from build123d import *

# Parameters (mm, degrees)
SKETCH3_W               = 130
SKETCH3_H               = 45
BOSS_EXTRUDE1_DEPTH     = 100
CUT_EXTRUDE1_DEPTH      = 122.372360939
CUT_EXTRUDE1_DEPTH_BACK = 122.372360939
BOSS_EXTRUDE2_DEPTH     = 8
CUT_EXTRUDE2_DEPTH      = 122.372360939
CUT_EXTRUDE2_DEPTH_BACK = 122.372360939
CUT_EXTRUDE3_DEPTH      = 122.372360939
CUT_EXTRUDE3_DEPTH_BACK = 122.372360939
CUT_EXTRUDE4_DEPTH      = 122.372360939
CUT_EXTRUDE4_DEPTH_BACK = 122.372360939
FILLET3_R               = 5
SKETCH16_R              = 10
SKETCH16_R_2            = 5
BOSS_EXTRUDE3_DEPTH     = 15
SKETCH19_R              = 6
CUT_EXTRUDE5_DEPTH      = 122.372360939
CUT_EXTRUDE6_DEPTH      = 147.735305908
CUT_EXTRUDE6_DEPTH_BACK = 147.735305908
SKETCH23_R              = 5
CUT_EXTRUDE7_DEPTH      = 15
CUT_EXTRUDE8_DEPTH      = 15
CUT_EXTRUDE9_DEPTH      = 166.548331311
CUT_EXTRUDE9_DEPTH_BACK = 166.548331311
SKETCH28_R              = 11


with BuildPart() as part:
    # Sketch3 → Boss-Extrude1 (new body)
    with BuildSketch(Plane(origin=(0, 0, 0), x_dir=(1, 0, 0), z_dir=(0, 1, 0))):
        Rectangle(SKETCH3_W, SKETCH3_H)
    extrude(amount=-BOSS_EXTRUDE1_DEPTH)

    # Sketch5 → Cut-Extrude1 (cut, two sides: drawn at the far end of the back side and taken through both)
    with BuildSketch(Plane.XY.offset(-CUT_EXTRUDE1_DEPTH_BACK)):
        Polygon((-65, 0), (-40, 0), (-40, -30), (-65, -60), align=None)
        Polygon((65, 0), (40, 0), (40, -30), (65, -60), align=None)
    extrude(amount=CUT_EXTRUDE1_DEPTH + CUT_EXTRUDE1_DEPTH_BACK, mode=Mode.SUBTRACT)

    # Sketch7 → Boss-Extrude2 (add)
    with BuildSketch(Plane(origin=(0, 0, 0), x_dir=(1, 0, 0), z_dir=(0, 1, 0))):
        with BuildLine():
            Line((-20, 15), (20, 15))
            ThreePointArc((20, 15), (35, 0), (20, -15))
            Line((20, -15), (-20, -15))
            ThreePointArc((-20, -15), (-35, 0), (-20, 15))
        make_face()
        with BuildLine():
            Line((-20, 10), (20, 10))
            ThreePointArc((20, 10), (30, 0), (20, -10))
            Line((20, -10), (-20, -10))
            ThreePointArc((-20, -10), (-30, 0), (-20, 10))
        make_face(mode=Mode.SUBTRACT)
    extrude(amount=BOSS_EXTRUDE2_DEPTH)

    # Sketch9 → Cut-Extrude2 (cut, two sides: drawn at the far end of the back side and taken through both)
    with BuildSketch(Plane.XY.offset(-CUT_EXTRUDE2_DEPTH_BACK)):
        Polygon((-30, -32.113231403), (-55, -62.113231403), (-55, -100), (55, -100), (55, -64.057510222), (30, -34.057510222), (30, -10), (-30, -10), align=None)
    extrude(amount=CUT_EXTRUDE2_DEPTH + CUT_EXTRUDE2_DEPTH_BACK, mode=Mode.SUBTRACT)

    # Sketch11 → Cut-Extrude3 (cut, two sides: drawn at the far end of the back side and taken through both)
    with BuildSketch(Plane(origin=(0, 0, 0), x_dir=(0, 0, -1), z_dir=(1, 0, 0)).offset(-CUT_EXTRUDE3_DEPTH_BACK)):
        with BuildLine():
            Line((-22.5, -100), (0, -100))
            ThreePointArc((0, -100), (-15.909902577, -93.409902577), (-22.5, -77.5))
            Line((-22.5, -77.5), (-22.5, -100))
        make_face()
    extrude(amount=CUT_EXTRUDE3_DEPTH + CUT_EXTRUDE3_DEPTH_BACK, mode=Mode.SUBTRACT)

    # Sketch12 → Cut-Extrude4 (cut, two sides: drawn at the far end of the back side and taken through both)
    with BuildSketch(Plane(origin=(0, 0, 0), x_dir=(0, 0, -1), z_dir=(1, 0, 0)).offset(-CUT_EXTRUDE4_DEPTH_BACK)):
        with BuildLine():
            Line((22.5, -100), (22.5, -77.5))
            ThreePointArc((22.5, -77.5), (15.909902577, -93.409902577), (0, -100))
            Line((0, -100), (22.5, -100))
        make_face()
    extrude(amount=CUT_EXTRUDE4_DEPTH + CUT_EXTRUDE4_DEPTH_BACK, mode=Mode.SUBTRACT)

    # Fillet3
    fillet3_edges = [part.edges().sort_by_distance(p)[0] for p in [
        (-40, 0, 0),
        (40, 0, 0),
    ]]
    fillet(fillet3_edges, radius=FILLET3_R - 0.0001)  # a hair under: the kernel refuses the full size

    # Sketch16 → Boss-Extrude3 (add)
    # profile 1 of 4: a face of its own
    with BuildSketch(Plane(origin=(40, 0, 0), x_dir=(0, 0, -1), z_dir=(1, 0, 0))):
        with Locations((0, -20)):
            Circle(SKETCH16_R)
        with Locations((0, -20)):
            Circle(SKETCH16_R_2, mode=Mode.SUBTRACT)
    # profile 2 of 4: a face of its own
    with BuildSketch(Plane(origin=(40, 0, 0), x_dir=(0, 0, -1), z_dir=(1, 0, 0))):
        with BuildLine():
            Line((1.3e-08, -30), (6.111197294, -30))
            Line((6.111197294, -30), (6.111197294, -27.915381711))
            ThreePointArc((6.111197294, -27.915381711), (3.228481297, -29.464507833), (1.3e-08, -30))
        make_face()
    # profile 3 of 4: a face of its own
    with BuildSketch(Plane(origin=(40, 0, 0), x_dir=(0, 0, -1), z_dir=(1, 0, 0))):
        with BuildLine():
            Line((-6.111197294, -27.915381711), (-6.111197294, -30))
            Line((-6.111197294, -30), (1.3e-08, -30))
            ThreePointArc((1.3e-08, -30), (-3.228481284, -29.464507837), (-6.111197294, -27.915381711))
        make_face()
    # profile 4 of 4: a face of its own
    with BuildSketch(Plane(origin=(40, 0, 0), x_dir=(0, 0, -1), z_dir=(1, 0, 0))):
        Polygon((-6.111197294, -30), (-6.111197294, -48.004109964), (6.111197294, -48.004109964), (6.111197294, -30), (1.3e-08, -30), align=None)
    boss_extrude3 = extrude(amount=BOSS_EXTRUDE3_DEPTH)

    # Mirror4: Boss-Extrude3 across plane
    add(boss_extrude3.mirror(Plane(origin=(0, 0, 0), x_dir=(0, 0, 1), z_dir=(1, 0, 0))))

    # Sketch19 → Cut-Extrude5 (cut, through all)
    with BuildSketch(Plane(origin=(0, 0, 0), x_dir=(1, 0, 0), z_dir=(0, 1, 0))):
        with Locations(Location((0, 0, 0), (0, 0, 270))):
            Circle(SKETCH19_R)
    extrude(amount=-CUT_EXTRUDE5_DEPTH, mode=Mode.SUBTRACT)

    # Sketch23 → Cut-Extrude6 (cut, two sides: drawn at the far end of the back side and taken through both)
    with BuildSketch(Plane(origin=(40, 0, 0), x_dir=(0, 0, -1), z_dir=(1, 0, 0)).offset(-CUT_EXTRUDE6_DEPTH_BACK)):
        with Locations((0, -20)):
            Circle(SKETCH23_R)
    extrude(amount=CUT_EXTRUDE6_DEPTH + CUT_EXTRUDE6_DEPTH_BACK, mode=Mode.SUBTRACT)

    # Sketch26 → Cut-Extrude7 (cut)
    with BuildSketch(Plane.XY.offset(6.111197294)):
        Polygon((-40, -44.113231403), (-40, -48.004109964), (-43.2423988, -48.004109964), align=None)
    extrude(amount=-CUT_EXTRUDE7_DEPTH, mode=Mode.SUBTRACT)

    # Sketch27 → Cut-Extrude8 (cut)
    with BuildSketch(Plane.XY.offset(6.111197294)):
        Polygon((40, -46.057510222), (40, -48.004109964), (41.622166452, -48.004109964), align=None)
    extrude(amount=-CUT_EXTRUDE8_DEPTH, mode=Mode.SUBTRACT)

    # Sketch28 → Cut-Extrude9 (cut, two sides: drawn at the far end of the back side and taken through both)
    with BuildSketch(Plane(origin=(65, 0, 0), x_dir=(0, 0, -1), z_dir=(1, 0, 0)).offset(-CUT_EXTRUDE9_DEPTH_BACK)):
        with Locations((0, -77.5)):
            Circle(SKETCH28_R)
    extrude(amount=CUT_EXTRUDE9_DEPTH + CUT_EXTRUDE9_DEPTH_BACK, mode=Mode.SUBTRACT)


solid = part.part
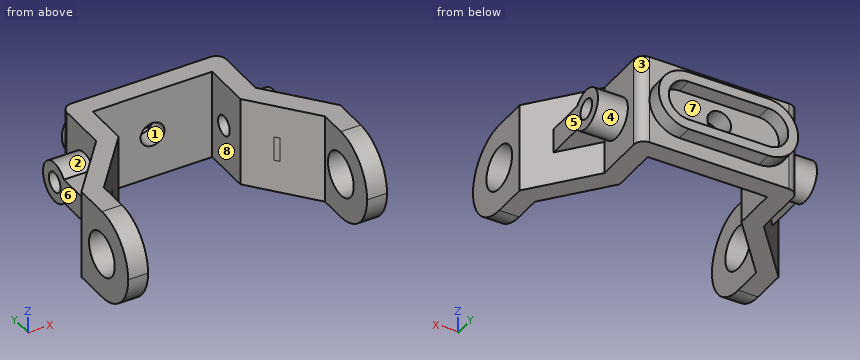
Design review of the part built by this model. Coordinates are the model's own, in mm. Face numbers are marked on the shaded views. A direction names the side the tool comes from. Give positions to 0.01 mm unless a question says otherwise; leave off trailing zeros. Write each loop counter-clockwise with the first axis right and the second up, starting at its lowest first coordinate (ties: lowest second). Pieces come first, ordered by that corner, then holes. Notation, with made-up numbers: M 7.5,-22.5 L 37.5,-22.5 A25 ccw 37.5,-1.5 Z; hole C -18,40 d3. An arc over 180 degrees is marked long. Answer as a JSON object with one key per item and string values. Group by question number.
1) Tool access review of the marked faces 4, 5, 6, 7 and 8: name each direction out of +Z, -Z, +X, -X, +Y, -Y from which nothing blocks a thin tool from reaching the whole face with its end or side.
2) We need section C-C (y = -90). Give the boundary of the cut face in (x, z), and give its area (3 significant figures).
3) We need section B-B (x = 33). Give the boundary of the cut face in (y, z), and give its area (3 significant figures).
4) Mouldability with a two-part tool opening along Y and no side actions: class the marked faces 1, 2 and 3 as released by +Y, released by -Y, zero draft, split by the parting line, or undercut.
5) We need section A-A (y = -20). Give the boundary of the cut face in (x, z).
6) Clearance check with flat-ended pins moving along their axes: pin 1 Ø5 at (y, z) = (-46.5, -16) entering from +X; pin 2 Ø6.5 at (x, y) = (-8.5, 4.5) entering from -Z; pin 3 Ø12 at (x, z) = (-50.5, 17) entering from -Y. State where each tip first meets the part, or that it passes through.
7) For line 1 along X through (y, z) = (-15.5, -16.5); line 2 along Z through (x, y) = (62.75, -77.5); line 3 along Z through (x, y) = (46.75, -20), list the stretches that pass through material, from the lowest coordinate up.
8) We need section D-D (z = 16.5). Give the boundary of the cut face in (x, y).
Answer key:
{
 "1": {"face 4": "+X", "face 5": "+Z, -Z, +X, +Y", "face 6": "+Z, -Z, -X, +Y", "face 7": "+Y", "face 8": "+Z, -Z, -Y"},
 "2": {"outline": "M -65,-18.71 L -55,-18.71 L -55,18.71 L -65,18.71 Z; M 55,-18.71 L 65,-18.71 L 65,18.71 L 55,18.71 Z", "area": "748 mm²"},
 "3": {"outline": "M -37.66,-22.5 L 0,-22.5 L 0,-7.48 L 8,-7.48 L 8,7.48 L 0,7.48 L 0,22.5 L -37.66,22.5 Z; hole C -20,0 d10", "area": "1,740 mm²"},
 "4": {"face 1": "zero draft", "face 2": "undercut", "face 3": "released by +Y"},
 "5": {"outline": "M -55,-10 L -40,-10 L -40,-22.5 L -30,-22.5 L -30,-5 L -55,-5 Z; M -55,5 L -30,5 L -30,22.5 L -40,22.5 L -40,10 L -55,10 Z; M 30,-22.5 L 40,-22.5 L 40,-10 L 55,-10 L 55,-5 L 30,-5 Z; M 30,5 L 55,5 L 55,10 L 40,10 L 40,22.5 L 30,22.5 Z"},
 "6": {"pin 1": "stops at x = 55.83", "pin 2": "stops at z = -15", "pin 3": "stops at y = -95.84"},
 "7": {"line 1": "x = -40 to -30, 30 to 40", "line 2": "z = -22.5 to -11, 11 to 22.5", "line 3": "z = -10 to -5, 5 to 10"},
 "8": {"outline": "M -65,-92.8 L -55,-92.8 L -55,-62.11 L -30,-32.11 L -30,-10 L 30,-10 L 30,-34.06 L 55,-64.06 L 55,-92.8 L 65,-92.8 L 65,-60 L 40,-30 L 40,-5 A5 ccw 35,0 L -35,0 A5 ccw -40,-5 L -40,-30 L -65,-60 Z"}
}
